Autodesk Inventor part; units mm, degrees
ref_plane "YZ Plane" through (0, 0, 0) normal (1, 0, 0) x (0, 1, 0)
ref_plane "XZ Plane" through (0, 0, 0) normal (0, 1, 0) x (-1, 0, 0)
ref_plane "XY Plane" through (0, 0, 0) normal (0, 0, 1) x (1, 0, 0)
sketch "Sketch1" plane through (0, 0, 0) normal (0, 1, 0) x (-1, 0, 0)
  line L0 (0, 0) -> (62.484, 0)
  line L1 (62.484, 0) -> (62.484, -90.932)
  line L2 (62.484, -90.932) -> (0, -90.932)
  line L3 (0, -90.932) -> (0, 0)
  dimension "d0" = 62.484
  dimension "d1" = 90.932
extrude "Extrusion1" add sketch "Sketch1" along normal blind 4.318
sketch "Sketch3" plane through (0, 0, 0) normal (0, -1, 0) x (1, 0, 0)
  line L0 (0, 0) -> (0, -90.932)
  line L1 (-62.484, -90.932) -> (-62.484, 0)
  line L2 (-62.484, 0) -> (0, 0)
  line L3 (0, -90.932) -> (-62.484, -90.932)
  line L4 (-9.017, -23.241) -> (-53.467, -23.241)
  line L5 (-53.467, -23.241) -> (-53.467, -67.691)
  line L6 (-53.467, -67.691) -> (-9.017, -67.691)
  line L7 (-9.017, -67.691) -> (-9.017, -23.241)
  line L8 (-9.017, -23.241) -> (-53.467, -67.691) construction
  line L9 (-53.467, -23.241) -> (-9.017, -67.691) construction
  point P0 (-31.242, -45.466)
  dimension "d13" = 44.45
  dimension "d14" = 44.45
extrude "Extrusion2" add sketch "Sketch3" along normal blind 6.35 contours L7 L6 L5 L4
sketch "Sketch2" plane through (0, 4.318, 0) normal (0, 1, 0) x (1, 0, 0)
  line L0 (-62.484, 90.932) -> (-62.484, 0)
  line L1 (-62.484, 45.466) -> (0, 45.466)
  line L2 (0, 90.932) -> (-62.484, 90.932)
  line L3 (-31.242, 90.932) -> (-31.242, 0)
  line L4 (-62.484, 0) -> (0, 0)
  line L5 (-18.542, 32.766) -> (-43.942, 32.766)
  line L6 (-43.942, 32.766) -> (-43.942, 58.166)
  line L7 (-43.942, 58.166) -> (-18.542, 58.166)
  line L8 (-18.542, 58.166) -> (-18.542, 32.766)
  line L9 (-18.542, 32.766) -> (-43.942, 58.166) construction
  line L10 (-43.942, 32.766) -> (-18.542, 58.166) construction
  point P0 (-31.242, 45.466)
  dimension "d4" = 25.4
  dimension "d5" = 25.4
hole "Hole1" at (-18.542, 4.318, -32.766) at (-43.942, 4.318, -32.766) at (-18.542, 4.318, -58.166) at (-43.942, 4.318, -58.166) direction (0, -1, 0) diameter 6.7564 depth 25.4 tip angle 118 countersink diameter 12.8778 countersink angle 82
fillet "Fillet1" radius 3.175 8 edges at (-31.242, 0, -23.241) (-31.242, -6.35, -23.241) (-31.242, -6.35, -67.691) (-31.242, 0, -67.691) (-9.017, 0, -45.466) (-53.467, 0, -45.466) (-53.467, -6.35, -45.466) (-9.017, -6.35, -45.466)
properties part number "caster adapter for mobile afl"
The listing builds one solid part. Answer for the finished solid, in the listing's coordinates (mm). Give positions to 0.01 mm unless a question says otherwise; leave off trailing zeros. Loops run counter-clockwise (first coordinate to the right, second up) from the corner with the lowest first, then second, coordinate; pieces in that order, holes last.
Item 1: Find the intervals of material crossed by line 1 along Z through (x, y) = (-40.5, 2.75); line 2 along Z through (x, y) = (-41, -4); line 3 along Y through (x, z) = (-33, -84), in increasing order.
Derived:
line 1: z = -90.93 to -61.9, -54.44 to -36.5, -29.04 to 0
line 2: z = -67.58 to -59.83, -56.51 to -34.43, -31.11 to -23.35
line 3: y = 0 to 4.32
Item 2: A cutting plane is placed at D-D (x = -45.5). Give the number of separate pieces and of enclosed holes in the cut face, then the cut area to 3 significant figures.
Derived:
separate pieces: 3
enclosed holes: 0
area: 524 mm2
Item 3: Determine the mould class of faces 1 (the flat face through (-31, 4.318, -45)), 2 (the cylindrical face through (-54.422, -0.905, -45.822)), 3 (the conical face through (-22, 1, -59)) for opening direction X: +X half, -X half, draft (parallel to the pull), parting line (faces both ways), or undercut.
Derived:
face 1: draft
face 2: -X half
face 3: undercut
Item 4: Each of these flat-tipped pins is pushed along its axis until it touches: pin 1 Ø8 at (x, z) = (-43.942, -58.166) entering from +Y; pin 2 Ø1.5 at (x, y) = (-30.5, -3) entering from -Z; pin 3 Ø1.5 at (y, z) = (0.5, -11) entering from +X; pin 4 Ø3 at (x, y) = (-11, -5) entering from +Z. Where does it stop, or does it pass through?
Derived:
pin 1: stops at y = 1.51
pin 2: stops at z = -67.83
pin 3: stops at x = 0
pin 4: stops at z = -23.26
Item 5: A cutting plane is placed at C-C (y = -5). Give the vertices of the cut face in (x, z).
Derived:
outline: (-52.89, -67.11) - (-9.59, -67.11) - (-9.59, -23.82) - (-52.89, -23.82) - close; hole circle Ø6.76 at (-43.94, -58.17); hole circle Ø6.76 at (-43.94, -32.77); hole circle Ø6.76 at (-18.54, -58.17); hole circle Ø6.76 at (-18.54, -32.77)
